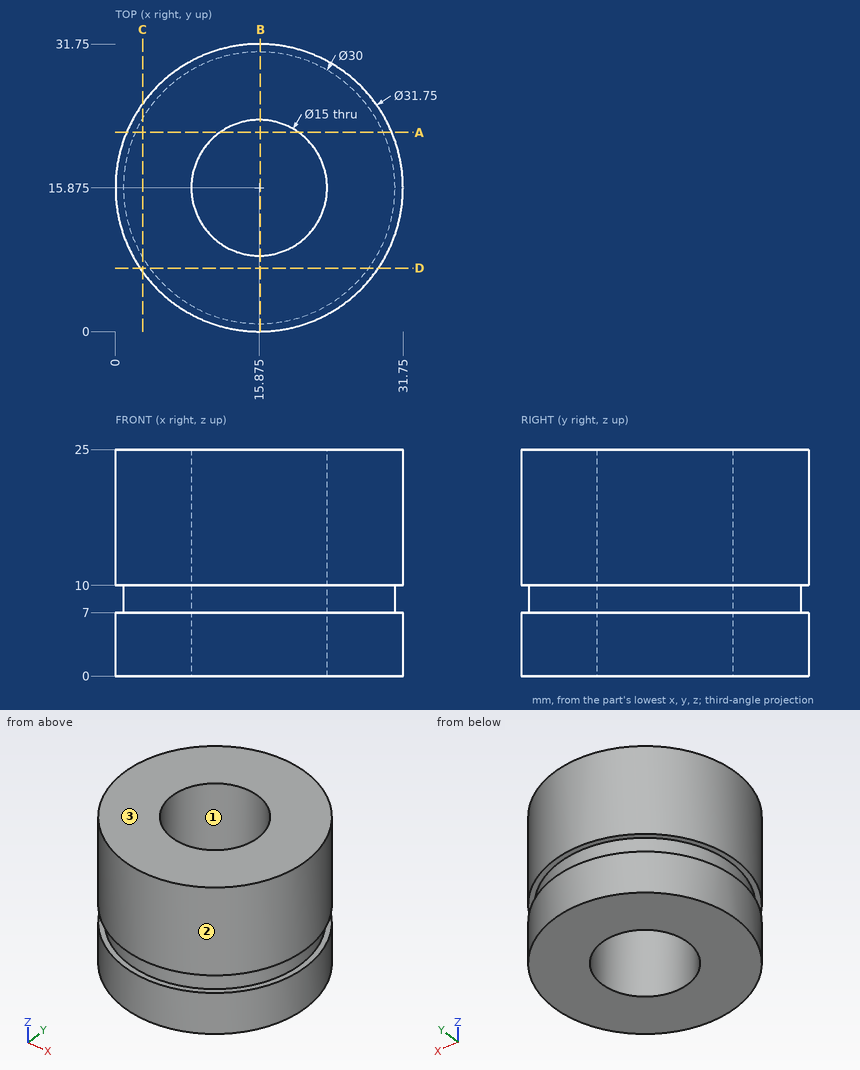
Geometry check sheet. Reference: drawing and pictorial views, mm from the part's lowest x, y, z. Give positions to 0.01 mm unless a question says otherwise; leave off trailing zeros. Loops run counter-clockwise (first coordinate to the right, second up) from the corner with the lowest first, then second, coordinate; pieces in that order, holes last. Notation, with made-up numbers: M 87,-6 L 100,-6 A8 cw 100,-1 Z; hole C 6,85 d4. An arc over 180 degrees is marked long. Use a Markdown table: item, result. Add a question column.
Q1. Scan lines: line 1 along X through (y, z) = (15.5, 17.75); line 2 along X through (y, z) = (10, 7.5); line 3 along Y through (x, z) = (10.5, 14). Record each from-to range of solid material in increasing order. Write a range as [from, to].
Q2. Sectioned sample at B-B, the plane x = 16. Record the cut outline in (y, z), then the cut area to 3 significant figures.
Q3. Sectioned sample at A-A, the plane y = 22. Record the cut outline in (x, z).
Q4. Sectioned sample at D-D, the plane y = 7. Record the cut outline in (x, z).
Q5. Mould release check, pull along Y, two halves, no side actions. Record for the marked faces 1, 2 and 3: pulls with the +Y half, pulls with the -Y half, needs draft (parallel to the pull), parting line crosses it, or undercut.
Q6. Sectioned sample at C-C, the plane x = 3. Record the cut outline in (y, z), then the cut area to 3 significant figures.
Q7. Go/stop test with flat-tipped pins: pin 1 (1 mm diameter, centred on y = 18.5, z = 6.5, fed in from +X); pin 2 (2 mm diameter, centred on y = 4, z = 4.5, fed in from -X); pin 3 (12 mm diameter, centred on y = 23.5, z = 9.5, fed in from -X). Record where each tip stops, or that it passes through.
Verdict:
| question | item | result |
|---|---|---|
| 1 | line 1 | [0, 8.38], [23.37, 31.75] |
| 1 | line 2 | [2.07, 11.21], [20.54, 29.68] |
| 1 | line 3 | [0.94, 10.64], [21.11, 30.81] |
| 2 | outline | M 0,0 L 8.38,0 L 8.38,25 L 0,25 L 0,10 L 0.88,10 L 0.88,7 L 0,7 Z; M 23.37,0 L 31.75,0 L 31.75,7 L 30.87,7 L 30.87,10 L 31.75,10 L 31.75,25 L 23.37,25 Z |
| 2 | area | 414 mm^2 |
| 3 | outline | M 1.23,0 L 11.55,0 L 11.55,25 L 1.23,25 L 1.23,10 L 2.18,10 L 2.18,7 L 1.23,7 Z; M 20.2,0 L 30.52,0 L 30.52,7 L 29.57,7 L 29.57,10 L 30.52,10 L 30.52,25 L 20.2,25 Z |
| 4 | outline | M 2.71,0 L 29.04,0 L 29.04,7 L 27.97,7 L 27.97,10 L 29.04,10 L 29.04,25 L 2.71,25 L 2.71,10 L 3.78,10 L 3.78,7 L 2.71,7 Z |
| 5 | face 1 | undercut |
| 5 | face 2 | parting line crosses it |
| 5 | face 3 | needs draft |
| 6 | outline | M 6.59,0 L 25.16,0 L 25.16,7 L 23.57,7 L 23.57,10 L 25.16,10 L 25.16,25 L 6.59,25 L 6.59,10 L 8.18,10 L 8.18,7 L 6.59,7 Z |
| 6 | area | 455 mm^2 |
| 7 | pin 1 | x = 31.61 |
| 7 | pin 2 | x = 4.31 |
| 7 | pin 3 | x = 0.09 |
